```python
from build123d import *

# Parameters (mm, degrees)
F0_W     = 25.4
F0_H     = 25.4
F1_DEPTH = 25.4
F2_SIZE  = 7.62
F3_W     = 10.16
F3_H     = 10.16
F4_DEPTH = 25.4


with BuildPart() as f1:
    # F0 (on Top) → F1 (new body)
    with BuildSketch(Plane.XY):
        with Locations((-12.7, -12.7)):
            Rectangle(F0_W, F0_H)
    extrude(amount=F1_DEPTH)

    # F2
    f2_edges = [f1.edges().sort_by_distance(p)[0] for p in [
        (-12.7, -25.4, 25.4),
        (-25.4, -12.7, 25.4),
        (-12.7, 0, 25.4),
        (0, -12.7, 25.4),
    ]]
    chamfer(f2_edges, length=F2_SIZE)

    # F3 (on face) → F4 (join)
    with BuildSketch(Plane.XY.offset(25.4)):
        with Locations((-12.7, -12.7)):
            Rectangle(F3_W, F3_H)
    extrude(amount=F4_DEPTH)


solid = f1.part
```
Input: part model. Units: mm. Frame: model coordinates. A direction names the side the tool comes from. Coordinates: 2 decimals unless noted, no trailing zeros. Write each loop counter-clockwise with the first axis right and the second up, starting at its lowest first coordinate (ties: lowest second). Pieces come first, ordered by that corner, then holes. Notation, with made-up numbers: (-20.5, 7) -> (11.5, 7) arc R27 ccw to (11.5, 26) -> close; hole circle Ø5 at (-38, -18.5). An arc over 180 degrees is marked (long way). Answer as a JSON object with one key per item and string values.
1. Section B-B on y = -18.5. Return the cut outline in (x, z), then the cut area to 3 significant figures.
Result set:
{"outline": "(-25.4, 0) -> (0, 0) -> (0, 17.78) -> (-6.9, 24.68) -> (-18.5, 24.68) -> (-25.4, 17.78) -> close", "area": "579 mm2"}
2. First-contact query: P1, Ø5, axis at y = -14, z = 37.5, coming from the -X side; P2, Ø5, axis at x = -12, z = 39, coming from the +Y side; P3, Ø4, axis at x = -13.5, z = 21, coming from the +Y side; P4, Ø6, axis at x = -21.5, z = 35, coming from the +Y side. Flat tips, straight axial feed; report the tip coordinate or a pass-through.
Result set:
{"P1": "stops at x = -17.78", "P2": "stops at y = -7.62", "P3": "stops at y = -1.22", "P4": "passes through"}
3. Access query for faces 1 (the face through (0, -13, 9)), 2 (the face through (-13, -17.78, 38)), 3 (the face through (-7.62, -13, 38)), 4 (the face through (-17.78, -13, 38)), 5 (the face through (-13, -7.62, 38)). Directions: +Z, -Z, +X, -X, +Y, -Y. A direction counts if a zero-diameter tool reaches every point of the face in a straight line with its end or side. Return the directions, or none.
Result set:
{"face 1": "+Z, -Z, +X, +Y, -Y", "face 2": "+Z, +X, -X, -Y", "face 3": "+Z, +X, +Y, -Y", "face 4": "+Z, -X, +Y, -Y", "face 5": "+Z, +X, -X, +Y"}
4. Section C-C on z = 20. Return the cut outline in (x, y), then the cut area to 3 significant figures.
Result set:
{"outline": "(-23.18, -23.18) -> (-2.22, -23.18) -> (-2.22, -2.22) -> (-23.18, -2.22) -> close", "area": "439 mm2"}
5. Section A-A on x = -13. Return the cut outline in (y, z), then the cut area to 3 significant figures.
Result set:
{"outline": "(-25.4, 0) -> (0, 0) -> (0, 17.78) -> (-7.62, 25.4) -> (-7.62, 50.8) -> (-17.78, 50.8) -> (-17.78, 25.4) -> (-25.4, 17.78) -> close", "area": "845 mm2"}
6. Material intervals for line 1 (Z direction, x = -18.75, y = -14.75); line 2 (Y direction, x = -13.25, z = 39); line 3 (Z direction, x = -6, y = -2.25), sorted ascending. Write a range as from..to.
Result set:
{"line 1": "z = 0..24.43", "line 2": "y = -17.78..-7.62", "line 3": "z = 0..20.03"}
